from build123d import *

# Parameters (mm, degrees)
BOSS_EXTRU_1_DEPTH = 5


with BuildPart() as part:
    # Esquisse1 → Boss.-Extru.1 (new body)
    with BuildSketch(Plane.XY):
        with BuildLine():
            Line((100, 145.707319285), (100, 240.707319285))
            Line((100, 240.707319285), (100, 275.707319285))
            Line((100, 275.707319285), (95, 275.707319285))
            Line((95, 275.707319285), (95, 315.707319285))
            Line((95, 315.707319285), (100, 315.707319285))
            Line((100, 315.707319285), (100, 450.707319285))
            ThreePointArc((100, 450.707319285), (42.075716698, 423.773030355), (0, 375.707319285))
            Line((0, 375.707319285), (0, 275.707319285))
            Line((0, 275.707319285), (5, 275.707319285))
            Line((5, 275.707319285), (5, 235.707319285))
            Line((5, 235.707319285), (0, 235.707319285))
            Line((0, 235.707319285), (0, 145.707319285))
            Line((0, 145.707319285), (40, 145.707319285))
            Line((40, 145.707319285), (40, 140.707319285))
            Line((40, 140.707319285), (60, 140.707319285))
            Line((60, 140.707319285), (60, 145.707319285))
            Line((60, 145.707319285), (100, 145.707319285))
        make_face()
    extrude(amount=BOSS_EXTRU_1_DEPTH)


solid = part.part
Input: part model. Units: mm. Frame: model coordinates. A direction names the side the tool comes from. Round coordinates to 2 decimals unless told otherwise and drop trailing zeros. Order: outer loops, then holes, each group sorted by start corner. A loop starts at its lowest first (then second) coordinate and runs counter-clockwise, first axis right, second up. Notation, with made-up numbers: (75, -2.75) - (134, -2.75) arc R21 ccw to (134, 17.25) - close; hole circle Ø7 at (66.25, 63). An arc over 180 degrees is marked (long way). Answer as a JSON object with one key per item and string values. Group by question number.
(1) Material intervals for probe 1 along X at (y, z) = (254, 1.1); probe 2 along Y at (x, z) = (4, 2.75); probe 3 along X at (y, z) = (436, 3.25), sorted ascending. Write a range as from..to.
(2) Reachability of faces 5 (the face through (97, 315.707, 2)), 6 (the face through (80, 145.707, 2)), 7 (the face through (5, 256, 2)), 8 (the face through (40, 143, 2)) from +Z, -Z, +X, -X, +Y, -Y: full face, straight path, thin tool, end or side. Return the list, or none.
(3) Cut plane B-B (y = 305.5). Return loops of the section in (x, z), then the cut area to 3 significant figures.
(4) Cut plane A-A (z = 2.05). Return loops of the section in (x, y), then the cut area to 3 significant figures.
(5) Cut plane C-C (x = 70.5). Return loops of the section in (y, z).
(6) Draft query along Y for faces 1 (the face through (20, 145.707, 2)), 2 (the face through (0, 191, 2)), 3 (the face through (42.798, 424.311, 2.465)), 4 (the face through (2, 275.707, 2)). Return one class per face: released by +Y, released by -Y, zero draft, split by the parting line, or undercut.
(7) Pin query (flat end, axial travel): P1, Ø2.5, axis at x = 1.5, z = 1.5, coming from the -Y side; P2, Ø2.5, axis at x = 97.5, z = 2.5, coming from the +Y side; P3, Ø1.5, axis at y = 314, z = 4, coming from the +X side. Return the tip coordinate at first contact, or that it passes through.
Here are the results:
{
 "1": {"probe 1": "x = 5..100", "probe 2": "y = 145.71..235.71, 275.71..382.44", "probe 3": "x = 61.15..100"},
 "2": {"face 5": "+Z, -Z, +X", "face 6": "+Z, -Z, +X, -Y", "face 7": "+Z, -Z, -X", "face 8": "+Z, -Z, -X, -Y"},
 "3": {"outline": "(0, 0) - (95, 0) - (95, 5) - (0, 5) - close", "area": "475 mm^2"},
 "4": {"outline": "(0, 145.71) - (40, 145.71) - (40, 140.71) - (60, 140.71) - (60, 145.71) - (100, 145.71) - (100, 275.71) - (95, 275.71) - (95, 315.71) - (100, 315.71) - (100, 450.71) arc R154.49 ccw to (0, 375.71) - (0, 275.71) - (5, 275.71) - (5, 235.71) - (0, 235.71) - close", "area": "27,600 mm^2"},
 "5": {"outline": "(145.71, 0) - (440.67, 0) - (440.67, 5) - (145.71, 5) - close"},
 "6": {"face 1": "released by -Y", "face 2": "zero draft", "face 3": "released by +Y", "face 4": "undercut"},
 "7": {"P1": "stops at y = 145.71", "P2": "stops at y = 450.41", "P3": "stops at x = 95"}
}
